Part model, mm, in its own coordinate system. A direction names the side the tool comes from. Round coordinates to 2 decimals unless told otherwise and drop trailing zeros. Write each loop counter-clockwise with the first axis right and the second up, starting at its lowest first coordinate (ties: lowest second). Pieces come first, ordered by that corner, then holes. Notation, with made-up numbers: M 41,-8.5 L 75,-8.5 A25 cw 75,18.5 Z; hole C -25,42.5 d9. An arc over 180 degrees is marked long. Use a Markdown table: item, result. Add a question column.
1) Which spindle directions (+Z, -Z, +X, -X, +Y, -Y) get a long thin tool onto all of the face, cutting with end or side? Do faces 4 (the face through (-44.934, -10.14, -7.294)), 5 (the face through (35, -15, 0)). Say none if no direction does.
2) Slice it at C-C on x = -40. Write the cut outline in (y, z).
3) Drop flat-ended pins along their axis: P1, Ø3, axis at y = -10.5, z = -4, coming from the -X side; P2, Ø6, axis at x = 40, z = 0, coming from the -Y side; P3, Ø5, axis at y = -16, z = -6.5, coming from the +X side; P4, Ø3, axis at x = -40, z = 0, coming from the -Y side. Give the stop position or say it passes through.
4) Slice it at D-D on y = -4.25. Write the cut outline in (x, z), plus the area to 3 significant figures.
5) Slice it at A-A on z = 0. Write the cut outline in (x, y), plus the area to 3 significant figures.
6) Wall check: probe 1 along X at (y, z) = (-2.5, 0); probe 2 along X at (y, z) = (-6.25, 0); probe 3 along X at (y, z) = (-18, 3.5). Give the ranges that are in metal, low to high.
7) Two-plate mould, pull along X, no slides. Class faces 1 (the face through (47.5, -10, 0)), 2 (the face through (0, -9, 0)), 3 (the face through (-30, 0, 0)): released by +X, released by -X, zero draft, split by the parting line, or undercut.
8) Slice it at B-B on y = -18. Write the cut outline in (x, z), plus the area to 3 significant figures.
```python
from build123d import *

# Parameters (mm, degrees)
SKETCH_W        = 95
SKETCH_H        = 20
SKETCH_R        = 2.6
PAD_DEPTH       = 20
SKETCH001_R     = 12
POCKET_DEPTH    = 20.001
SKETCH002_R     = 5
POCKET001_DEPTH = 10
FILLET_R        = 9


with BuildPart() as part:
    # Sketch → Pad (new body)
    with BuildSketch(Plane.XZ):
        Rectangle(SKETCH_W, SKETCH_H)
        with Locations((-40, 0)):
            Circle(SKETCH_R, mode=Mode.SUBTRACT)
        with Locations((40, 0)):
            Circle(SKETCH_R, mode=Mode.SUBTRACT)
    extrude(amount=PAD_DEPTH)

    # Sketch001 (on Face2 of Pad) → Pocket (cut, through all)
    with BuildSketch(Plane.XY.offset(10)):
        with Locations((0, 3)):
            Circle(SKETCH001_R)
    extrude(amount=-POCKET_DEPTH, mode=Mode.SUBTRACT)

    # Sketch002 (on Face5 of Pocket) → Pocket001 (cut)
    with BuildSketch(Plane.XZ.offset(20)):
        with Locations((-40, 0)):
            Circle(SKETCH002_R)
        with Locations((40, 0)):
            Circle(SKETCH002_R)
    extrude(amount=-POCKET001_DEPTH, mode=Mode.SUBTRACT)

    # Fillet
    fillet_edges = [part.edges().sort_by_distance(p)[0] for p in [
        (-47.5, -10, 10),
        (-47.5, -10, -10),
        (47.5, -10, 10),
        (47.5, -10, -10),
    ]]
    fillet(fillet_edges, radius=FILLET_R)


solid = part.part
```
Entries:
| question | item | result |
|---|---|---|
| 1 | face 4 | -Z, -X, +Y, -Y |
| 1 | face 5 | -Y |
| 2 | outline | M -20,-9.87 L 0,-9.87 L 0,-2.6 L -10,-2.6 L -10,-5 L -20,-5 Z; M -20,5 L -10,5 L -10,2.6 L 0,2.6 L 0,9.87 L -20,9.87 Z |
| 3 | P1 | stops at x = -47.37 |
| 3 | P2 | stops at y = -10 |
| 3 | P3 | stops at x = 46.99 |
| 3 | P4 | passes through |
| 4 | outline | M -47.5,-1 A9 ccw -38.5,-10 L -9.56,-10 L -9.56,10 L -38.5,10 A9 ccw -47.5,1 Z; M 9.56,-10 L 38.5,-10 A9 ccw 47.5,-1 L 47.5,1 A9 ccw 38.5,10 L 9.56,10 Z; hole C -40,0 d5.2; hole C 40,0 d5.2 |
| 4 | area | 1,410 mm^2 |
| 5 | outline | M -47.5,-20 L -45,-20 L -45,-10 L -42.6,-10 L -42.6,0 L -47.5,0 Z; M -37.4,-10 L -35,-10 L -35,-20 L 35,-20 L 35,-10 L 37.4,-10 L 37.4,0 L 11.62,0 A12 cw -11.62,0 L -37.4,0 Z; M 42.6,-10 L 45,-10 L 45,-20 L 47.5,-20 L 47.5,0 L 42.6,0 Z |
| 5 | area | 1,440 mm^2 |
| 6 | probe 1 | x = -47.5 to -42.6, -37.4 to -10.67, 10.67 to 37.4, 42.6 to 47.5 |
| 6 | probe 2 | x = -47.5 to -42.6, -37.4 to -7.64, 7.64 to 37.4, 42.6 to 47.5 |
| 6 | probe 3 | x = -47.15 to -43.57, -36.43 to 36.43, 43.57 to 47.15 |
| 7 | face 1 | released by +X |
| 7 | face 2 | undercut |
| 7 | face 3 | zero draft |
| 8 | outline | M -47.5,-1 A9 ccw -38.5,-10 L 38.5,-10 A9 ccw 47.5,-1 L 47.5,1 A9 ccw 38.5,10 L -38.5,10 A9 ccw -47.5,1 Z; hole C -40,0 d10; hole C 40,0 d10 |
| 8 | area | 1,670 mm^2 |
